Work out the finished part from the listing and answer in its coordinate system (mm). A direction names the side the tool comes from. Round coordinates to 2 decimals unless told otherwise and drop trailing zeros. Write each loop counter-clockwise with the first axis right and the second up, starting at its lowest first coordinate (ties: lowest second). Pieces come first, ordered by that corner, then holes.
1. Find section A-A (y = -17.5). Write down the section's boundary in (x, z).
2. A flat-ended cylindrical pin translates along its axis: pin 1 Ø6 at (x, y) = (0, 17.5) entering from +Z. Find the tip coordinate at first contact, or state that the pin passes through.
3. A tool of negligible diameter and unlimited length cuts with its end or side. For faces 5 (the face through (15, 0, 4)), 6 (the face through (-5.642, -5.776, 0.304)), 7 (the face through (-5, 6, 4)), from which of +Z, -Z, +X, -X, +Y, -Y can it reach the whole face along a straight path? Write none if from no direction.
4. Find section C-C (x = 0). Write down the section's boundary in (y, z).
5. Straight lines are drawn through the part: probe 1 along Y at (x, z) = (0, 6.25); probe 2 along Y at (x, z) = (8, 7); probe 3 along Y at (x, z) = (1.25, 0.5). For each, find the intervals that lie inside material, in ascending order.
6. Determine the mould class of faces 1 (the face through (-0.011, -10.586, 4.248)), 2 (the face through (0, 27, 4)), 3 (the face through (5, -6, 4)), 4 (the face through (-7, 6, 0)) for opening direction Y: pulls with the +Y half, pulls with the -Y half, needs draft (parallel to the pull), parting line crosses it, or undercut.
7. Find section B-B (z = 1.25). Write down the section's boundary in (x, y).
8. Find section D-D (x = -7.75). Write down the section's boundary in (y, z).
```python
from build123d import *

# Parameters (mm, degrees)
SKETCH1_W            = 30
SKETCH1_H            = 54
BOSS_EXTRUDE1_DEPTH  = 8
M4_CLEARANCE_HOLE1_D = 4.8
CUT_EXTRUDE1_REACH   = 33.906
FILLET1_R            = 1
CHAMFER1_SIZE        = 0.6


with BuildPart() as part:
    # Sketch1 → Boss-Extrude1 (new body)
    with BuildSketch(Plane.XY):
        Rectangle(SKETCH1_W, SKETCH1_H)
    extrude(amount=BOSS_EXTRUDE1_DEPTH)

    # M4 Clearance Hole1 (through all)
    with Locations(Plane.XY.offset(8)):
        with Locations((0, 17.5), (0, -17.5)):
            Hole(M4_CLEARANCE_HOLE1_D / 2)

    # Sketch4 → Cut-Extrude1 (cut, up to next)
    with BuildSketch(Plane.XY.offset(8), mode=Mode.PRIVATE) as cut_extrude1_sk1:
        Polygon((11, 0), (0, 11), (-11, 0), (0, -11), align=None)
    cut_extrude1_tool1 = extrude(cut_extrude1_sk1.sketch, amount=-CUT_EXTRUDE1_REACH, mode=Mode.PRIVATE) & part.part
    add(cut_extrude1_tool1.solids().sort_by_distance((0, 0, 8))[0], mode=Mode.SUBTRACT)

    # Fillet1
    fillet1_edges = [part.edges().sort_by_distance(p)[0] for p in [
        (11, 0, 4),
        (0, -11, 4),
        (-11, 0, 4),
        (0, 11, 4),
        (-15, 27, 4),
        (15, 27, 4),
        (15, -27, 4),
        (-15, -27, 4),
    ]]
    fillet(fillet1_edges, radius=FILLET1_R)

    # Chamfer1
    chamfer1_edges = [part.edges().sort_by_distance(p)[0] for p in [
        (2.4, -17.5, 0),
        (2.4, 17.5, 0),
        (5.5, -5.5, 0),
        (-5.5, -5.5, 0),
        (5.5, 5.5, 0),
        (-5.5, 5.5, 0),
        (15, 0, 0),
        (-15, 0, 0),
        (0, 27, 0),
        (0, -27, 0),
        (-14.707106781, 26.707106781, 0),
        (14.707106781, 26.707106781, 0),
        (-14.707106781, -26.707106781, 0),
        (14.707106781, -26.707106781, 0),
        (0, -10.585786438, 0),
        (10.585786438, 0, 0),
        (0, 10.585786438, 0),
        (-10.585786438, 0, 0),
    ]]
    chamfer(chamfer1_edges, length=CHAMFER1_SIZE)


solid = part.part
```
Worked answers:
1. outline: (-15, 0.6) - (-14.4, 0) - (-3, 0) - (-2.4, 0.6) - (-2.4, 8) - (-15, 8) - close; (2.4, 0.6) - (3, 0) - (14.4, 0) - (15, 0.6) - (15, 8) - (2.4, 8) - close
2. pin 1: stops at z = 8
3. face 5: +Z, -Z, +X, +Y, -Y
3. face 6: -Z
3. face 7: +Z, -Z
4. outline: (-27, 0.6) - (-26.4, 0) - (-20.5, 0) - (-19.9, 0.6) - (-19.9, 8) - (-27, 8) - close; (-15.1, 0.6) - (-14.5, 0) - (-11.19, 0) - (-10.59, 0.6) - (-10.59, 8) - (-15.1, 8) - close; (10.59, 0.6) - (11.19, 0) - (14.5, 0) - (15.1, 0.6) - (15.1, 8) - (10.59, 8) - close; (19.9, 0.6) - (20.5, 0) - (26.4, 0) - (27, 0.6) - (27, 8) - (19.9, 8) - close
5. probe 1: y = -27 to -19.9, -15.1 to -10.59, 10.59 to 15.1, 19.9 to 27
5. probe 2: y = -27 to -3, 3 to 27
5. probe 3: y = -26.9 to -19.67, -15.33 to -9.89, 9.89 to 15.33, 19.67 to 26.9
6. face 1: undercut
6. face 2: pulls with the +Y half
6. face 3: undercut
6. face 4: needs draft
7. outline: (-15, -26) arc R1 ccw to (-14, -27) - (14, -27) arc R1 ccw to (15, -26) - (15, 26) arc R1 ccw to (14, 27) - (-14, 27) arc R1 ccw to (-15, 26) - close; hole (-10.29, -0.71) - (-0.71, -10.29) arc R1 ccw to (0.71, -10.29) - (10.29, -0.71) arc R1 ccw to (10.29, 0.71) - (0.71, 10.29) arc R1 ccw to (-0.71, 10.29) - (-10.29, 0.71) arc R1 ccw to start; hole circle Ø4.8 at (0, -17.5); hole circle Ø4.8 at (0, 17.5)
8. outline: (-27, 0.6) - (-26.4, 0) - (-4.1, 0) - (-3.25, 0.6) - (-3.25, 8) - (-27, 8) - close; (3.25, 0.6) - (4.1, 0) - (26.4, 0) - (27, 0.6) - (27, 8) - (3.25, 8) - close
